The listing builds one solid part. Answer for the finished solid, in the listing's coordinates (mm). A direction names the side the tool comes from. Give positions to 0.01 mm unless a question says otherwise; leave off trailing zeros. Write each loop counter-clockwise with the first axis right and the second up, starting at its lowest first coordinate (ties: lowest second). Pieces come first, ordered by that corner, then holes.
```python
from build123d import *

# Parameters (mm, degrees)
F0_W   = 50.8
F0_H   = 33.506379
F0_W_2 = 76.2
F0_H_2 = 87.548942


with BuildPart() as f1:
    # F0 (on Right) → F1 (revolve)
    with BuildSketch(Plane.YZ):
        with Locations((-6.972096, 72.144307)):
            Rectangle(F0_W, F0_H)
        with Locations((1.404499, -5.676974)):
            Rectangle(F0_W_2, F0_H_2)
        Polygon((-32.372096, 55.391118), (-36.695501, 38.097497), (39.504499, 38.097497), (18.427904, 55.391118), align=None)
    revolve(axis=Axis((0, -36.695501, -5.676974), (0, 0, -1)))


solid = f1.part
```
Item 1: Which of the six approach directions +Z, -Z, +X, -X, +Y, -Y give full straight-line access (tool end or side, diameter ignored) to faces 1 (the face through (-46.367, -97.165, -5.064)), 2 (the face through (0.19, -41.015, 72.379))?
Conclusion:
face 1: +Z, -Z
face 2: +Z
Item 2: Each of these flat-tipped pins is pushed along its axis until it touches: P1, Ø3, axis at y = -54, z = 35, coming from the +X side; P2, Ø6, axis at y = -88.5, z = -25.5, coming from the +X side; P3, Ø2, axis at y = -12, z = 45, coming from the +X side. Where does it stop, or does it pass through?
Conclusion:
P1: stops at x = 74.54
P2: stops at x = 58.52
P3: stops at x = 64.49
Item 3: Consider probe 1 along X at (y, z) = (-79, 38); probe 2 along Y at (x, z) = (64, -17); probe 3 along Y at (x, z) = (41.5, -30.5). Determine where each line is inside the solid, lowest interval first.
Conclusion:
probe 1: x = -63.38 to 63.38
probe 2: y = -78.05 to 4.66
probe 3: y = -100.6 to 27.21
Item 4: Determine the mould class of faces 3 (the face through (0.094, -38.825, 46.623)), 4 (the face through (-11, -36, 88.897)), 5 (the face through (-53.81, -48.65, 72.38)) for opening direction Y: pulls with the +Y half, pulls with the -Y half, needs draft (parallel to the pull), parting line crosses it, or undercut.
Conclusion:
face 3: undercut
face 4: needs draft
face 5: parting line crosses it
Item 5: A cutting plane is placed at A-A, the plane z = 61. Give the vertices of the cut face in (x, y).
Conclusion:
outline: circle Ø110.25 at (0, -36.7); hole circle Ø8.65 at (0, -36.7)
Item 6: A cutting plane is placed at B-B, the plane z = -11. Give the vertices of the cut face in (x, y).
Conclusion:
outline: circle Ø152.4 at (0, -36.7)
